Input: part model. Units: mm. Frame: model coordinates. Face numbers are marked on the shaded views. A direction names the side the tool comes from. Coordinates: 2 decimals unless noted, no trailing zeros. Order: outer loops, then holes, each group sorted by start corner. A loop starts at its lowest first (then second) coordinate and runs counter-clockwise, first axis right, second up. Notation, with made-up numbers: (7, 45) - (29, 45) arc R16 cw to (29, 75) - close; hole circle Ø7 at (56.25, -21). An arc over 180 degrees is marked (long way). Answer as CSV lines item,"result". Start each with the question number.
Item 1: Section D-D (y = 14.5). Output: boundary loops of the cut face in (x, z), and give its area (3 significant figures).
Item 2: Material intervals for line 1 along X through (y, z) = (54, 0); line 2 along X through (y, z) = (13.5, 0); line 3 along Z through (x, y) = (-4.5, 56), sorted ascending.
Item 3: Access query for the marked faces 1 and 2. Directions: +Z, -Z, +X, -X, +Y, -Y. A direction counts if a zero-diameter tool reaches every point of the face in a straight line with its end or side. Return the directions, or none.
Item 4: Section C-C (y = 41). Output: boundary loops of the cut face in (x, z).
Item 5: First-contact query: pin 1 (2 mm diameter, centred on x = -11, z = -11, fed in from +Y); pin 2 (4 mm diameter, centred on x = -6.5, y = 51, fed in from -Z); pin 3 (8.5 mm diameter, centred on x = 1.5, z = 3.5, fed in from +Y); pin 4 (5 mm diameter, centred on y = 13.5, z = 10, fed in from +X). Flat tips, straight axial feed; report the tip coordinate or a pass-through.
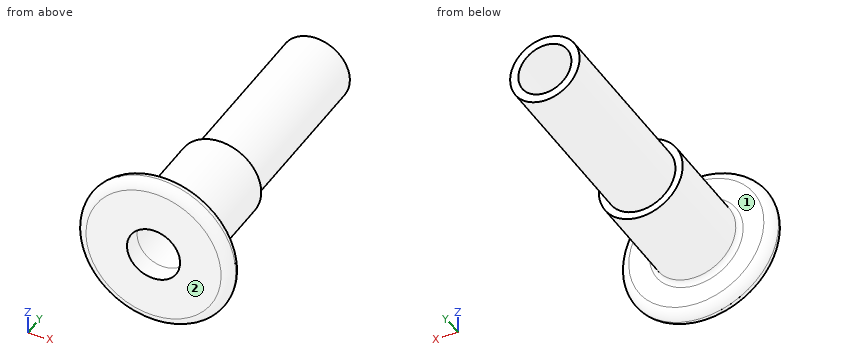
from build123d import *

# Parameters (mm, degrees)
SKETCH1_R           = 8.7
SKETCH1_R_2         = 5.5
BOSS_EXTRUDE1_DEPTH = 68.8
BOSS_EXTRUDE2_START = 4
SKETCH2_R           = 16
SKETCH2_R_2         = 5.5
BOSS_EXTRUDE2_DEPTH = 4
FILLET1_R           = 2
FILLET2_R           = 1
BOSS_EXTRUDE6_START = -10
BOSS_EXTRUDE6_DEPTH = 10
CUT_EXTRUDE1_START  = -23
SKETCH10_R          = 8.7
SKETCH10_R_2        = 7.2
CUT_EXTRUDE1_DEPTH  = 23
SKETCH11_R          = 17.428070689
CUT_EXTRUDE2_DEPTH  = 54.972215104
SKETCH12_R          = 7.2
SKETCH12_R_2        = 5.5
BOSS_EXTRUDE7_DEPTH = 14.9


with BuildPart() as part:
    # Sketch1 → Boss-Extrude1 (new body)
    with BuildSketch(Plane(origin=(0, 0, 0), x_dir=(1, 0, 0), z_dir=(0, 1, 0))):
        with Locations(Location((0, 0, 0), (0, 0, 90))):
            Circle(SKETCH1_R)
        with Locations(Location((0, 0, 0), (0, 0, 90))):
            Circle(SKETCH1_R_2, mode=Mode.SUBTRACT)
    extrude(amount=BOSS_EXTRUDE1_DEPTH)

    # Sketch2 → Boss-Extrude2 (add)
    with BuildSketch(Plane.XZ.offset(BOSS_EXTRUDE2_START)):
        with Locations(Location((0, 0, 0), (0, 0, 270))):
            Circle(SKETCH2_R)
        with Locations(Location((0, 0, 0), (0, 0, 270))):
            Circle(SKETCH2_R_2, mode=Mode.SUBTRACT)
    extrude(amount=-BOSS_EXTRUDE2_DEPTH)

    # Fillet1
    fillet1_edges = [part.edges().sort_by_distance(p)[0] for p in [
        (0, 0, 16),
        (0, -4, 16),
    ]]
    fillet(fillet1_edges, radius=FILLET1_R - 0.0001)  # a hair under: the kernel refuses the full size

    # Fillet2
    fillet2_edges = [part.edges().sort_by_distance(p)[0] for p in [
        (0, 0, 8.7),
    ]]
    fillet(fillet2_edges, radius=FILLET2_R)

    # Sketch7 → Boss-Extrude6 (add)
    with BuildSketch(Plane(origin=(0, 68.8, 0), x_dir=(1, 0, 0), z_dir=(0, 1, 0)).offset(BOSS_EXTRUDE6_START)):
        with BuildLine():
            Line((-8.459778344, -2.030307951), (-9.805994948, -2.807572454))
            ThreePointArc((-9.805994948, -2.807572454), (-8.832386986, -5.101856537), (-7.331446138, -7.091537035))
            Line((-7.331446138, -7.091537035), (-5.988187435, -6.311228981))
            ThreePointArc((-5.988187435, -6.311228981), (-7.534421013, -4.35), (-8.459778344, -2.030307951))
        make_face()
        with BuildLine():
            Line((-2.471590909, 8.341536931), (-2.475728155, 9.89498712))
            ThreePointArc((-2.475728155, 9.89498712), (0, 10.2), (2.475728155, 9.89498712))
            Line((2.475728155, 9.89498712), (2.471590909, 8.341536931))
            ThreePointArc((2.471590909, 8.341536931), (0, 8.7), (-2.471590909, 8.341536931))
        make_face()
        with BuildLine():
            Line((8.459778344, -2.030307951), (9.807174294, -2.803450085))
            ThreePointArc((9.807174294, -2.803450085), (8.833459119, -5.1), (7.331446138, -7.091537035))
            Line((7.331446138, -7.091537035), (5.988187435, -6.311228981))
            ThreePointArc((5.988187435, -6.311228981), (7.534421013, -4.35), (8.459778344, -2.030307951))
        make_face()
    extrude(amount=BOSS_EXTRUDE6_DEPTH)

    # Sketch10 → Cut-Extrude1 (cut)
    with BuildSketch(Plane(origin=(0, 45, 0), x_dir=(1, 0, 0), z_dir=(0, 1, 0)).offset(CUT_EXTRUDE1_START)):
        with Locations(Location((0, 0, 0), (0, 0, 90))):
            Circle(SKETCH10_R)
        with Locations(Location((0, 0, 0), (0, 0, 270))):
            Circle(SKETCH10_R_2, mode=Mode.SUBTRACT)
    extrude(amount=CUT_EXTRUDE1_DEPTH, mode=Mode.SUBTRACT)

    # Sketch11 → Cut-Extrude2 (cut, through all)
    with BuildSketch(Plane.XZ.offset(-45)):
        Circle(SKETCH11_R)
    extrude(amount=-CUT_EXTRUDE2_DEPTH, mode=Mode.SUBTRACT)

    # Sketch12 → Boss-Extrude7 (add)
    with BuildSketch(Plane(origin=(0, 45, 0), x_dir=(1, 0, 0), z_dir=(0, 1, 0))):
        with Locations(Location((0, 0, 0), (0, 0, 270))):
            Circle(SKETCH12_R)
        with Locations(Location((0, 0, 0), (0, 0, 90))):
            Circle(SKETCH12_R_2, mode=Mode.SUBTRACT)
    extrude(amount=BOSS_EXTRUDE7_DEPTH)


solid = part.part
Determined:
1,outline,"circle Ø17.4 at (0, 0); hole circle Ø11 at (0, 0)"
1,area,"143 mm^2"
2,line 1,"x = -7.2 to -5.5, 5.5 to 7.2"
2,line 2,"x = -8.7 to -5.5, 5.5 to 8.7"
2,line 3,"z = -5.62 to -3.16, 3.16 to 5.62"
3,face 1,"+Y"
3,face 2,"+Z, -Z, +X, -X, -Y"
4,outline,"circle Ø14.4 at (0, 0); hole circle Ø11 at (0, 0)"
5,pin 1,"stops at y = -0.08"
5,pin 2,"stops at z = -5.62"
5,pin 3,"stops at y = 59.9"
5,pin 4,"stops at x = 4.41"
